The model under review builds one solid part; all positions refer to its coordinate system, in mm. A direction names the side the tool comes from. Give positions to 0.01 mm unless a question says otherwise; leave off trailing zeros. Order: outer loops, then holes, each group sorted by start corner. A loop starts at its lowest first (then second) coordinate and runs counter-clockwise, first axis right, second up.
```python
from build123d import *

# Parameters (mm, degrees)
SKETCH_1_R          = 8.99
EXTRUDE_1_DEPTH     = 20
SKETCH_2_R          = 10
EXTRUDE_2_DEPTH     = 5
CHAMFER_1_SIZE      = 2
SKETCH_3_R          = 1.9
CUT_EXTRUDE_1_DEPTH = 36


with BuildPart() as part:
    # 草图1 → 凸台-拉伸1 (new body)
    with BuildSketch(Plane(origin=(0, 0, 0), x_dir=(1, 0, 0), z_dir=(0, 1, 0))):
        with Locations(Location((0, 0, 0), (0, 0, 270))):
            Circle(SKETCH_1_R)
    extrude(amount=EXTRUDE_1_DEPTH)

    # 草图2 → 凸台-拉伸2 (add)
    with BuildSketch(Plane(origin=(0, 20, 0), x_dir=(1, 0, 0), z_dir=(0, 1, 0))):
        with Locations(Location((0, 0, 0), (0, 0, 270))):
            Circle(SKETCH_2_R)
    extrude(amount=EXTRUDE_2_DEPTH)

    # 倒角1
    chamfer_1_edges = [part.edges().sort_by_distance(p)[0] for p in [
        (0, 0, -8.99),
    ]]
    chamfer(chamfer_1_edges, length=CHAMFER_1_SIZE)

    # 草图3 → 切除-拉伸1 (cut)
    with BuildSketch(Plane(origin=(0, 25, 0), x_dir=(1, 0, 0), z_dir=(0, 1, 0))):
        with Locations(Location((5, 0, 0), (0, 0, 270))):
            Circle(SKETCH_3_R)
        with Locations(Location((-2.5, -4.330127019, 0), (0, 0, 270))):
            Circle(SKETCH_3_R)
        with Locations(Location((-2.5, 4.330127019, 0), (0, 0, 270))):
            Circle(SKETCH_3_R)
    extrude(amount=-CUT_EXTRUDE_1_DEPTH, mode=Mode.SUBTRACT)

    # 草图5 → 切除-旋转1 (revolve, cut)
    with BuildSketch(Plane.XY, mode=Mode.PRIVATE) as cut_revolve_1_sk:
        Polygon((0, 23), (-2.5, 23), (-5.780837962, 26.280837962), (0, 26.280837962), align=None)
    revolve(cut_revolve_1_sk.sketch.rotate(Axis((0, 0, 0), (0, 1, 0)), 82.281327408), axis=Axis((0, 0, 0), (0, 1, 0)), mode=Mode.SUBTRACT)


solid = part.part
```
Item 1: For line 1 (X direction, y = 8.75, z = 0); line 2 (Z direction, x = -2.5, y = 16.25); line 3 (Z direction, x = -1, y = 16), list the stretches that pass through material, from the lowest coordinate up.
Values found:
line 1: x = -8.99 to 3.1, 6.9 to 8.99
line 2: z = -8.64 to -6.23, -2.43 to 2.43, 6.23 to 8.64
line 3: z = -8.93 to -5.5, -3.16 to 3.16, 5.5 to 8.93
Item 2: Take a section at B-B (x = 0). Give the boundary of the cut face in (y, z).
Values found:
outline: (0, -6.99) - (2, -8.99) - (20, -8.99) - (20, -10) - (25, -10) - (25, -4.5) - (23, -2.5) - (23, 2.5) - (25, 4.5) - (25, 10) - (20, 10) - (20, 8.99) - (2, 8.99) - (0, 6.99) - close
Item 3: Take a section at C-C (y = 16.5). Give the boundary of the cut face in (x, z).
Values found:
outline: circle Ø17.98 at (0, 0); hole circle Ø3.8 at (-2.5, -4.33); hole circle Ø3.8 at (-2.5, 4.33); hole circle Ø3.8 at (5, 0)
Item 4: For faces 4 (the flat face through (0, 23, 0)), 5 (the flat face through (2, 20, -9)), 6 (the cylindrical face through (6.602, 12.675, 1.021)), list the 3-axis set-ups (+Z, -Z, +X, -X, +Y, -Y) from which the entire face can be reached by the end or side of a thin tool; tool diameter is ignored.
Values found:
face 4: +Y
face 5: -Y
face 6: +Y, -Y
Item 5: Clearance check with flat-ended pins moving along their axes: pin 1 Ø8 at (x, y) = (4, 17) entering from +Z; pin 2 Ø6 at (y, z) = (8.5, 0) entering from +X; pin 3 Ø8 at (y, z) = (7.5, -6) entering from -X; pin 4 Ø3 at (x, z) = (-2.5, 4.33) entering from +Y. State where each tip first meets the part, or that it passes through.
Values found:
pin 1: stops at z = 9.91
pin 2: stops at x = 8.99
pin 3: stops at x = -8.76
pin 4: passes through
Item 6: Take a section at A-A (z = 0). Give the boundary of the cut face in (x, y).
Values found:
outline: (-10, 20) - (-8.99, 20) - (-8.99, 2) - (-6.99, 0) - (3.1, 0) - (3.1, 23.6) - (2.5, 23) - (-2.5, 23) - (-4.5, 25) - (-10, 25) - close; (6.9, 0) - (6.99, 0) - (8.99, 2) - (8.99, 20) - (10, 20) - (10, 25) - (6.9, 25) - close
Item 7: Draft analysis for pull direction X (two halves, no side actions). For faces 1 (the conical face through (-2.471, 23.125, 0.888)), 2 (the flat face through (-4.3, 25, 2.1)), 3 (the cylindrical face through (-9.76, 22.46, -2.17)), state which applies: released by +X, released by -X, zero draft, split by the parting line, or undercut.
Values found:
face 1: undercut
face 2: zero draft
face 3: split by the parting line
